Print and shaded views of the part. All mm, measured from the part's lowest x, y and z. A direction names the side the tool comes from. Round coordinates to 2 decimals unless told otherwise and drop trailing zeros. Write each loop counter-clockwise with the first axis right and the second up, starting at its lowest first coordinate (ties: lowest second). Pieces come first, ordered by that corner, then holes.
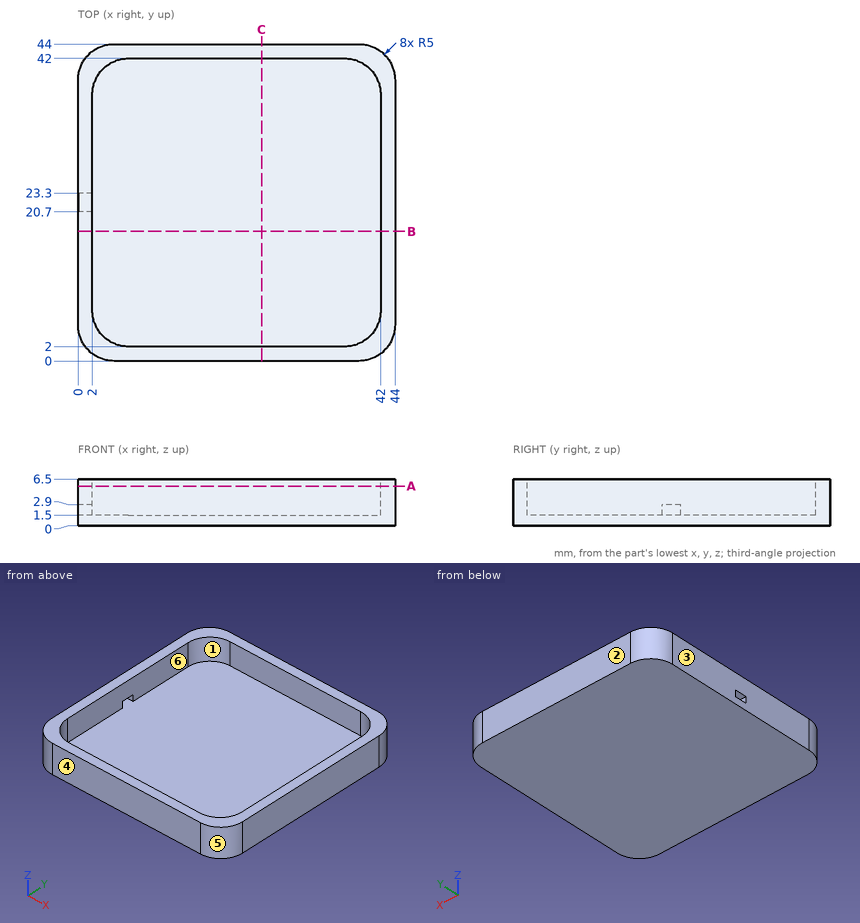
1) Wall check: L1, parallel to X at y = 17, z = 3.25; L2, parallel to Z at x = 12, y = 39. Give the ranges that are in metal, low to high.
Results:
L1: x = 0 to 2, 42 to 44
L2: z = 0 to 1.5
2) Mould opens along X. For the marked faces 3, 4, 5 and 6 say: released by +X, released by -X, zero draft, split by the parting line, or undercut.
Results:
face 3: released by -X
face 4: zero draft
face 5: released by +X
face 6: undercut
3) Slice it at A-A (z = 5.5). Write the cut outline in (x, y), plus the area to 3 significant figures.
Results:
outline: (0, 5) arc R5 ccw to (5, 0) - (39, 0) arc R5 ccw to (44, 5) - (44, 39) arc R5 ccw to (39, 44) - (5, 44) arc R5 ccw to (0, 39) - close; hole (2, 7) arc R5 ccw to (7, 2) - (37, 2) arc R5 ccw to (42, 7) - (42, 37) arc R5 ccw to (37, 42) - (7, 42) arc R5 ccw to (2, 37) - close
area: 336 mm2
4) Pin check, flat tips, straight feed: pin 1 Ø12 at (x, y) = (7, 25.5) entering from +Z; pin 2 Ø1.1 at (x, z) = (1, 2) entering from -Y; pin 3 Ø4 at (x, y) = (14, 15.5) entering from +Z; pin 4 Ø1.5 at (x, z) = (1.5, 2) entering from +Y. Stop position of each tip, or through.
Results:
pin 1: stops at z = 6.5
pin 2: stops at y = 1.38
pin 3: stops at z = 1.5
pin 4: stops at y = 43.18
5) Which spindle directions (+Z, -Z, +X, -X, +Y, -Y) get a long thin tool onto all of the face, cutting with end or side? Do the marked faces 1 and 2. Say none if no direction does.
Results:
face 1: +Z
face 2: +Z, -Z, +X, -X, +Y
6) Slice it at B-B (y = 18). Write the cut outline in (x, z), plus the area to 3 significant figures.
Results:
outline: (0, 0) - (44, 0) - (44, 6.5) - (42, 6.5) - (42, 1.5) - (2, 1.5) - (2, 6.5) - (0, 6.5) - close
area: 86.0 mm2
